```python
from build123d import *

# Parameters (mm, degrees)
SKETCH1_W           = 48
SKETCH1_H           = 77
BOSS_EXTRUDE1_DEPTH = 5
SKETCH2_R           = 1.2
BOSS_EXTRUDE2_DEPTH = 3
FILLET1_R           = 0.75
FILLET2_R           = 2
SKETCH3_R           = 8
CUT_EXTRUDE1_DEPTH  = 6


with BuildPart() as part:
    # Sketch1 → Boss-Extrude1 (new body)
    with BuildSketch(Plane(origin=(0, 0, 0), x_dir=(1, 0, 0), z_dir=(0, 1, 0))):
        with Locations((1.910432331, 3.349532818)):
            Rectangle(SKETCH1_W, SKETCH1_H)
    extrude(amount=BOSS_EXTRUDE1_DEPTH)

    # Sketch2 → Boss-Extrude2 (add)
    with BuildSketch(Plane(origin=(0, 5, 0), x_dir=(1, 0, 0), z_dir=(0, 1, 0))):
        with Locations((-19.839567669, 39.699532818)):
            Circle(SKETCH2_R)
        with Locations((23.660432331, 39.699532818)):
            Circle(SKETCH2_R)
        with Locations((23.660432331, -33.000467182)):
            Circle(SKETCH2_R)
        with Locations((-19.839567669, -33.000467182)):
            Circle(SKETCH2_R)
    extrude(amount=BOSS_EXTRUDE2_DEPTH)

    # Fillet1
    fillet1_edges = [part.edges().sort_by_distance(p)[0] for p in [
        (-21.039567669, 5, -39.699532818),
        (22.460432331, 5, -39.699532818),
        (22.460432331, 5, 33.000467182),
        (-21.039567669, 5, 33.000467182),
    ]]
    fillet(fillet1_edges, radius=FILLET1_R)

    # Fillet2
    fillet2_edges = [part.edges().sort_by_distance(p)[0] for p in [
        (-22.089567669, 2.5, -41.849532818),
        (25.910432331, 2.5, -41.849532818),
        (25.910432331, 2.5, 35.150467182),
        (-22.089567669, 2.5, 35.150467182),
    ]]
    fillet(fillet2_edges, radius=FILLET2_R)

    # Sketch3 → Cut-Extrude1 (cut, through all)
    with BuildSketch(Plane(origin=(0, 5, 0), x_dir=(1, 0, 0), z_dir=(0, 1, 0))):
        with Locations((1.910432331, 20.344226446)):
            Circle(SKETCH3_R)
        with Locations((1.910432331, -13.645160811)):
            Circle(SKETCH3_R)
    extrude(amount=-CUT_EXTRUDE1_DEPTH, mode=Mode.SUBTRACT)


solid = part.part
```
Part model, mm, in its own coordinate system. A direction names the side the tool comes from. Round coordinates to 2 decimals unless told otherwise and drop trailing zeros. Write each loop counter-clockwise with the first axis right and the second up, starting at its lowest first coordinate (ties: lowest second). Pieces come first, ordered by that corner, then holes.
Item 1: Cut at A-A, the plane z = 18.5. Give the cut face in (x, y).
Results:
outline: (-22.09, 0) - (-4.45, 0) - (-4.45, 5) - (-22.09, 5) - close; (8.27, 0) - (25.91, 0) - (25.91, 5) - (8.27, 5) - close
Item 2: Cut at C-C, the plane y = 4. Give the cut face in (x, z).
Results:
outline: (-22.09, -39.85) arc R2 ccw to (-20.09, -41.85) - (23.91, -41.85) arc R2 ccw to (25.91, -39.85) - (25.91, 33.15) arc R2 ccw to (23.91, 35.15) - (-20.09, 35.15) arc R2 ccw to (-22.09, 33.15) - close; hole circle Ø16 at (1.91, -20.34); hole circle Ø16 at (1.91, 13.65)
Item 3: Drop flat-ended pins along their axis: pin 1 Ø2 at (x, z) = (18, 0) entering from -Y; pin 2 Ø14.5 at (x, z) = (3, 12.5) entering from +Y; pin 3 Ø9.5 at (x, z) = (1.91, -20.34) entering from +Y (3 decimals). Give the stop position or say it passes through.
Results:
pin 1: stops at y = 0
pin 2: stops at y = 5
pin 3: passes through
Item 4: Which spindle directions (+Z, -Z, +X, -X, +Y, -Y) get a long thin tool onto all of the face, cutting with end or side? Do faces 1 (the cylindrical face through (24.214, 6.859, 34.065)), 2 (the flat face through (-20, 8, -40)). Say none if no direction does.
Results:
face 1: +Y
face 2: +Z, -Z, +X, -X, +Y
Item 5: Two-plate mould, pull along Z, no slides. Class faces 3 (the cylindrical face through (-21.52, 2.54, 34.55)), 4 (the cylindrical face through (24.805, 6.859, -40.06)), 5 (the flat face through (-22.09, 2, -3)), 6 (the flat face through (2, 2, -41.85)): +Z half, -Z half, draft (parallel to the pull), parting line (faces both ways), or undercut.
Results:
face 3: +Z half
face 4: undercut
face 5: draft
face 6: -Z half
Item 6: Probe L1, parallel to Z at x = 2, y = 1.5; L2, parallel to Z at x = 0.5, y = 1.75; L3, parallel to Y at x = 20.5, z = 29. List the from-to ranges inside material, lowest first.
Results:
L1: z = -41.85 to -28.34, -12.34 to 5.65, 21.64 to 35.15
L2: z = -41.85 to -28.22, -12.47 to 5.77, 21.52 to 35.15
L3: y = 0 to 5
Item 7: Cut at B-B, the plane x = 9. Give the cut face in (y, z), plus the area to 3 significant figures.
Results:
outline: (0, -41.85) - (5, -41.85) - (5, -24.05) - (0, -24.05) - close; (0, -16.64) - (5, -16.64) - (5, 9.94) - (0, 9.94) - close; (0, 17.35) - (5, 17.35) - (5, 35.15) - (0, 35.15) - close
area: 311 mm2
Item 8: Cut at D-D, the plane z = -35. Give the cut face in (x, y).
Results:
outline: (-22.09, 0) - (25.91, 0) - (25.91, 5) - (-22.09, 5) - close
